Check sheet for the modelled part. Datum: model origin and axes. Units: mm. Give positions to 0.01 mm unless a question says otherwise; leave off trailing zeros. Write each loop counter-clockwise with the first axis right and the second up, starting at its lowest first coordinate (ties: lowest second). Pieces come first, ordered by that corner, then holes. Notation, with made-up numbers: (53, 11) -> (105, 11) arc R21 ccw to (105, 41) -> close; hole circle Ø6 at (65.5, -35.75). An arc over 180 degrees is marked (long way). Answer as a JSON object with one key per item and string values.
from build123d import *

# Parameters (mm, degrees)
SKETCH_1_R      = 32
SKETCH_1_R_2    = 26
EXTRUDE_1_DEPTH = 13
FILLET_1_R      = 1.5


with BuildPart() as part:
    # 草图1 → 凸台-拉伸1 (new, symmetric)
    with BuildSketch(Plane(origin=(0, 0, 0), x_dir=(1, 0, 0), z_dir=(0, 1, 0))):
        with Locations(Location((0, 0, 0), (0, 0, 90))):
            Circle(SKETCH_1_R)
        with Locations(Location((0, 0, 0), (0, 0, 90))):
            Circle(SKETCH_1_R_2, mode=Mode.SUBTRACT)
    extrude(amount=EXTRUDE_1_DEPTH, both=True)

    # 草图2 → 旋转1 (revolve)
    with BuildSketch(Plane.XY, mode=Mode.PRIVATE) as revolve_1_sk:
        with BuildLine():
            Line((-32, 13), (-26, 13))
            ThreePointArc((-26, 13), (-29, 13.460607986), (-32, 13))
        make_face()
    revolve_1 = revolve(revolve_1_sk.sketch.rotate(Axis((0, 0, 0), (0, 1, 0)), 270), axis=Axis((0, 0, 0), (0, 1, 0)))

    # 镜向1: 旋转1 across plane
    add(revolve_1.mirror(Plane.ZX))

    # 圆角1
    fillet_1_edges = [part.edges().sort_by_distance(p)[0] for p in [
        (0, -13, 32),
        (0, 13, 32),
    ]]
    fillet(fillet_1_edges, radius=FILLET_1_R)


solid = part.part
1. Mould release check, pull along Z, two halves, no side actions. Record for faces 1 (the face through (15.821, -0.182, 20.633)), 2 (the face through (28.39, 0.166, -14.766)): released by +Z, released by -Z, zero draft, split by the parting line, or undercut.
Determined:
{"face 1": "undercut", "face 2": "split by the parting line"}
2. Scan lines: L1, parallel to X at y = -0.5, z = 0; L2, parallel to Z at x = 15.5, y = 10.25; L3, parallel to Z at x = -1.5, y = 10. Record each from-to range of solid material in increasing order. Write a range as [from, to].
Determined:
{"L1": "[-32, -26], [26, 32]", "L2": "[-28, -20.87], [20.87, 28]", "L3": "[-31.96, -25.96], [25.96, 31.96]"}
3. Go/stop test with flat-tipped pins: P1, Ø6, axis at x = -5.5, y = -9.5, coming from the -Z side; P2, Ø6, axis at x = 2, z = -24.5, coming from the -Y side; P3, Ø8, axis at y = -2.5, z = 21, coming from the +X side. Record where each tip stops, or that it passes through.
Determined:
{"P1": "z = -31.9", "P2": "y = -13.36", "P3": "x = 27.11"}
4. Sectioned sample at A-A, the plane y = 5.75. Enter the section's corners in (x, z), plus the area to 3 significant figures.
Determined:
{"outline": "circle Ø64 at (0, 0); hole circle Ø52 at (0, 0)", "area": "1,090 mm^2"}
